Could you check a few things on this drawing? It's one solid part, dimensions in mm from its lowest x, y, z. A direction names the side the tool comes from. Give positions to 0.01 mm unless a question says otherwise; leave off trailing zeros. Loops run counter-clockwise (first coordinate to the right, second up) from the corner with the lowest first, then second, coordinate; pieces in that order, holes last. Notation, with made-up numbers: M 29,32.25 L 50,32.25 A29 ccw 50,68.25 Z; hole C 36.25,37.25 d4. An arc over 180 degrees is marked long. One line per item, written item: value. Start each with the question number.
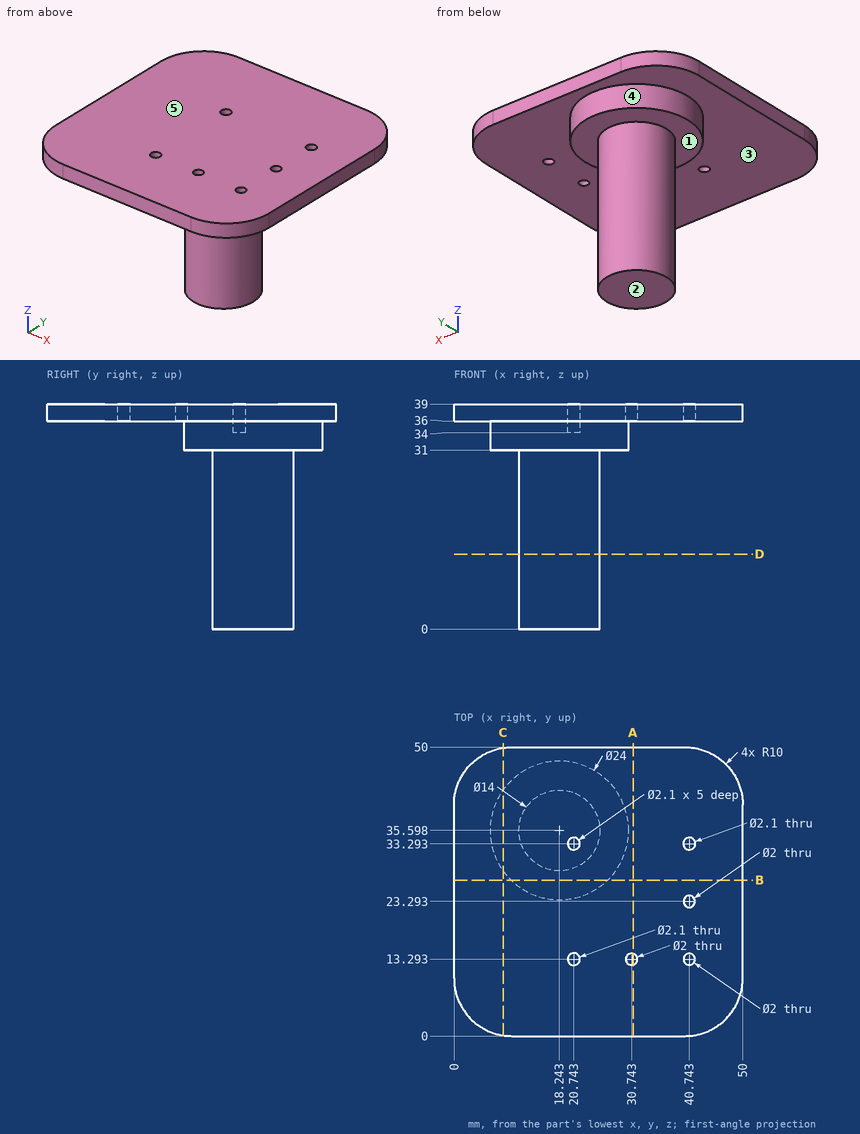
Q1. Which directions (+Z, -Z, +X, -X, +Y, -Y) give clear straight access to the entire face, cutting with the end or side of a thin tool? Please do the marked faces 1 and 2.
Q2. If we section it at B-B, the plane y = 27: Write out the boundary of the cut face in (x, z), plus the area to 3 significant figures.
Q3. If we mould it in two halves opening along Z, with no side actions, what happens to the marked faces 3, 4 and 5? For each: released by +Z, released by -Z, zero draft, split by the parting line, or undercut.
Q4. If we section it at C-C, the plane x = 8.5: Write out the boundary of the cut face in (y, z).
Q5. If we section it at A-A, the plane x = 31: Write out the boundary of the cut face in (y, z).
Q6. If we section it at D-D, the plane z = 13: Write out the boundary of the cut face in (x, y).
Q7. For P1, Ø15, axis at x = 19, y = 15.5, coming from the -Z side; P2, Ø5, axis at y = 43, z = 14, coming from the +X side; P3, Ø1.9, axis at x = 20.74, y = 33.29, coming from the -Z side; P4, Ø1.7, axis at x = 20.74, y = 13.29, coming from the -Z side, each with a flat end and sliding along its axis, tell me the tip position at first contact or that it passes through.
Q8. I need wall thicknesses on line 1 along Z through (x, y) = (11.5, 6); line 2 along Z through (x, y) = (28.5, 40); line 3 along Y through (x, z) = (31.5, 36.5) (1 decimal). Which ranges of each line are inside material? Lowest first, please.
Response:
1. face 1: -Z
1. face 2: -Z, +X, -X, +Y, -Y
2. outline: M 0,36 L 9.87,36 L 9.87,31 L 26.61,31 L 26.61,36 L 50,36 L 50,39 L 0,39 Z
2. area: 234 mm^2
3. face 3: released by -Z
3. face 4: zero draft
3. face 5: released by +Z
4. outline: M 0.11,36 L 28.59,36 L 28.59,31 L 42.6,31 L 42.6,36 L 49.89,36 L 49.89,39 L 0.11,39 Z
5. outline: M 0,36 L 12.33,36 L 12.33,39 L 0,39 Z; M 14.26,36 L 50,36 L 50,39 L 14.26,39 Z
6. outline: C 18.24,35.6 d14
7. P1: z = 36
7. P2: x = 23.24
7. P3: z = 0
7. P4: through
8. line 1: 36 to 39
8. line 2: 31 to 39
8. line 3: 0 to 12.6, 13.9 to 50
